Geometry check sheet. Reference: the model listing, model coordinates, mm. A direction names the side the tool comes from. Round coordinates to 2 decimals unless told otherwise and drop trailing zeros. Write item = value, one per line.
```python
from build123d import *

# Parameters (mm, degrees)
F0_R     = 14.2875
F0_R_2   = 9.525
F1_DEPTH = 12.7
F2_R     = 17.65
F2_R_2   = 9.525
F3_DEPTH = 4.75
F4_SIZE  = 0.5


with BuildPart() as f1:
    # F0 (on Top) → F1 (new body)
    with BuildSketch(Plane.XY):
        Circle(F0_R)
        Circle(F0_R_2, mode=Mode.SUBTRACT)
    extrude(amount=-F1_DEPTH)

    # F2 (on Top) → F3 (join)
    with BuildSketch(Plane.XY):
        Circle(F2_R)
        Circle(F2_R_2, mode=Mode.SUBTRACT)
    extrude(amount=F3_DEPTH)

    # F4
    f4_edges = [f1.edges().sort_by_distance(p)[0] for p in [
        (17.65, 0, 2.375),
        (-17.65, 0, 0),
        (-17.65, 0, 4.75),
        (9.525, 0, -6.35),
        (-9.525, 0, 0),
        (-9.525, 0, -12.7),
        (14.2875, 0, -6.35),
        (-14.2875, 0, 0),
        (-14.2875, 0, -12.7),
    ]]
    chamfer(f4_edges, length=F4_SIZE)


solid = f1.part
```
(1) Set-up check for faces 4 (the flat face through (8, 13, 0)), 5 (the cylindrical face through (-14.006, -10.74, 2.349)): record each of +Z, -Z, +X, -X, +Y, -Y from which the full face is reachable in a straight line by a thin tool's end or side.
Answers follow:
face_4 = -Z
face_5 = +Z, -Z
(2) Mould release check, pull along Y, two halves, no side actions. Record for faces 1 (the cylindrical face through (-14.274, 0.628, -6.268)), 2 (the cylindrical face through (-7.559, -5.796, -4.09)), 3 (the flat face through (0.96, -10.15, -12.7)): pulls with the +Y half, pulls with the -Y half, needs draft (parallel to the pull), parting line crosses it, or undercut.
Answers follow:
face_1 = parting line crosses it
face_2 = undercut
face_3 = needs draft
(3) Gauge pin test, flat ends, axial feed: pin 1 (10 mm diameter, centred on x = -13, z = -6, fed in from +Y); pin 2 (4 mm diameter, centred on y = -3.5, z = -9, fed in from -X); pin 3 (2 mm diameter, centred on y = 8.5, z = -2, fed in from -X). Record the tip position at first contact, or that the pin passes through.
Answers follow:
pin_1 = 11.84
pin_2 = -14.21
pin_3 = -12.16
(4) Scan lines: L1, parallel to Z at x = -1.5, y = 15; L2, parallel to X at y = 1, z = -1; L3, parallel to Y at x = 0.5, z = -5. Record each from-to range of solid material in increasing order. Write a range as [from, to].
Answers follow:
L1 = [0, 4.75]
L2 = [-14.25, -9.47], [9.47, 14.25]
L3 = [-14.28, -9.51], [9.51, 14.28]
